Job drawing, mm, ordinate dimensions from the low corner. One solid piece. Give positions to 0.01 mm unless a question says otherwise; leave off trailing zeros. Loops run counter-clockwise (first coordinate to the right, second up) from the corner with the lowest first, then second, coordinate; pieces in that order, holes last. Notation, with made-up numbers: M 40,1.5 L 62,1.5 A20 cw 62,37.5 Z; hole C -29,85.25 d2. An arc over 180 degrees is marked long. Put each result on its own line as item: value.
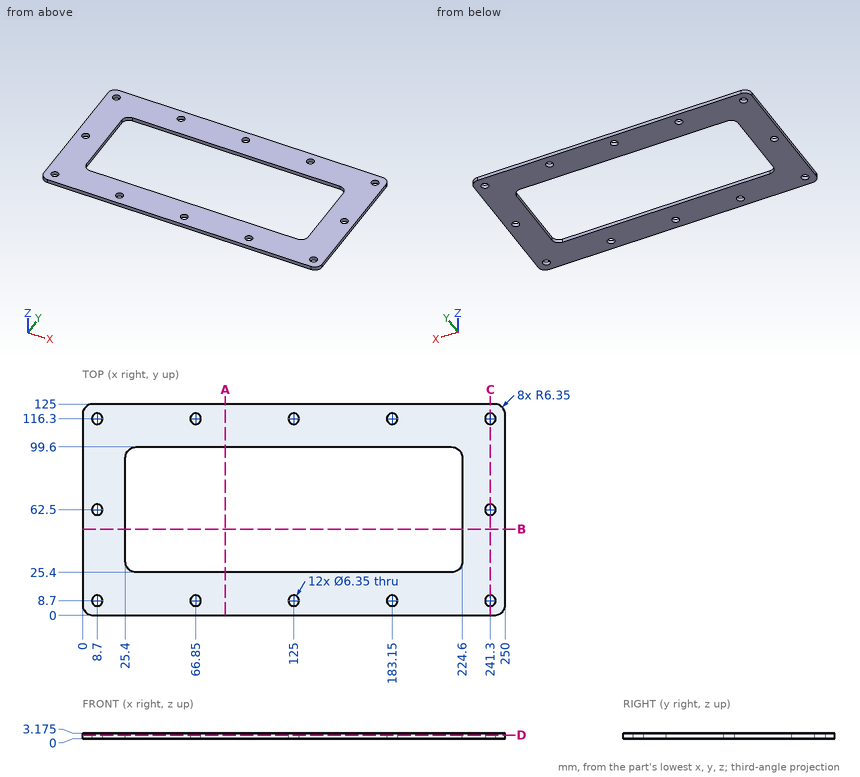
Q1. Slice it at D-D (z = 2.15). State how many separate pieces and enclosed holes the cut face has, and give its area (3 significant figures).
Here are the results:
separate pieces: 1
enclosed holes: 13
area: 16,100 mm²
Q2. Slice it at B-B (y = 51). List the corners of the cut face in (x, z) (3 decimals), and give its area (3 significant figures).
Here are the results:
outline: M 0,0 L 25.4,0 L 25.4,3.175 L 0,3.175 Z; M 224.6,0 L 250,0 L 250,3.175 L 224.6,3.175 Z
area: 161 mm²
Q3. Slice it at C-C (x = 241.3). List the corners of the cut face in (y, z) (3 decimals).
Here are the results:
outline: M 0,0 L 5.525,0 L 5.525,3.175 L 0,3.175 Z; M 11.875,0 L 59.325,0 L 59.325,3.175 L 11.875,3.175 Z; M 65.675,0 L 113.125,0 L 113.125,3.175 L 65.675,3.175 Z; M 119.475,0 L 125,0 L 125,3.175 L 119.475,3.175 Z
Q4. Slice it at A-A (x = 84.5). List the corners of the cut face in (y, z) (3 decimals).
Here are the results:
outline: M 0,0 L 25.4,0 L 25.4,3.175 L 0,3.175 Z; M 99.6,0 L 125,0 L 125,3.175 L 99.6,3.175 Z
Q5. Probe line 1 (Y direction, x = 196, z = 0.9); line 2 (X direction, y = 50, z = 1.2); line 3 (X direction, y = 8, z = 0.95). List the from-to ranges inside material, lowest first. Write a range as from..to.
Here are the results:
line 1: 0..25.4, 99.6..125
line 2: 0..25.4, 224.6..250
line 3: 0..5.6, 11.8..63.75, 69.95..121.9, 128.1..180.05, 186.25..238.2, 244.4..250
